Could you check a few things on this model? Use its own coordinates, in mm. Give positions to 0.01 mm unless a question says otherwise; leave off trailing zeros. Loops run counter-clockwise (first coordinate to the right, second up) from the corner with the lowest first, then second, coordinate; pieces in that order, holes last.
1. Imagine slicing it at C-C (x = -2.5). List the corners of the cut face in (y, z) for me, plus the area to 3 significant figures.
2. Imagine slicing it at A-A (x = 0). List the corners of the cut face in (y, z) for me (3 decimals), plus the area to 3 significant figures.
3. Imagine slicing it at B-B (y = 0). List the corners of the cut face in (x, z) for me.
4. For P1, Ø1.7, axis at x = 1.5, y = 0, coming from the -Z side; P2, Ø3, axis at y = -4, z = 3, coming from the -X side; P3, Ø3, axis at x = -2, z = 1.5, coming from the +Y side, each with a flat end and sliding along its axis, tell me the tip position at first contact or that it passes through.
5. I need wall thicknesses on line 1 along X through (y, z) = (0, 2.25); line 2 along X through (y, z) = (3, 12); line 3 along Z through (x, y) = (1.75, -1.5). Which ranges of each line are inside material? Lowest first, please.
```python
from build123d import *

# Parameters (mm, degrees)
F0_R     = 6.35
F1_DEPTH = 12.7
F2_W     = 1.27
F2_H     = 0.508
F2_W_2   = 0.508
F2_H_2   = 1.27
F3_DEPTH = 12.7
F4_R     = 0.254
F6_DEPTH = 10.16
F7_R     = 3.302
F8_DEPTH = 3.175


with BuildPart() as f1:
    # F0 (on Top) → F1 (new body)
    with BuildSketch(Plane.XY):
        Circle(F0_R)
    extrude(amount=F1_DEPTH)

    # F2 (on Top) → F3 (join, through all)
    with BuildSketch(Plane.XY):
        with Locations((0, 6.57217)):
            Rectangle(F2_W, F2_H)
        Polygon((-2.025599, 6.549563), (-3.198926, 6.063555), (-3.004523, 5.594224), (-1.831196, 6.080232), align=None)
        Polygon((-4.377818, 5.275844), (-5.275844, 4.377818), (-4.916634, 4.018608), (-4.018608, 4.916634), align=None)
        Polygon((-6.063555, 3.198926), (-6.549563, 2.025599), (-6.080232, 1.831196), (-5.594224, 3.004523), align=None)
        with Locations((-6.57217, 0)):
            Rectangle(F2_W_2, F2_H_2)
        Polygon((-6.549563, -2.025599), (-6.063555, -3.198926), (-5.594224, -3.004523), (-6.080232, -1.831196), align=None)
        Polygon((-5.275844, -4.377818), (-4.377818, -5.275844), (-4.018608, -4.916634), (-4.916634, -4.018608), align=None)
        Polygon((-3.198926, -6.063555), (-2.025599, -6.549563), (-1.831196, -6.080232), (-3.004523, -5.594224), align=None)
        with Locations((0, -6.57217)):
            Rectangle(F2_W, F2_H)
        Polygon((2.025599, -6.549563), (3.198926, -6.063555), (3.004523, -5.594224), (1.831196, -6.080232), align=None)
        Polygon((4.377818, -5.275844), (5.275844, -4.377818), (4.916634, -4.018608), (4.018608, -4.916634), align=None)
        Polygon((6.063555, -3.198926), (6.549563, -2.025599), (6.080232, -1.831196), (5.594224, -3.004523), align=None)
        with Locations((6.57217, 0)):
            Rectangle(F2_W_2, F2_H_2)
        Polygon((6.549563, 2.025599), (6.063555, 3.198926), (5.594224, 3.004523), (6.080232, 1.831196), align=None)
        Polygon((5.275844, 4.377818), (4.377818, 5.275844), (4.018608, 4.916634), (4.916634, 4.018608), align=None)
        Polygon((3.198926, 6.063555), (2.025599, 6.549563), (1.831196, 6.080232), (3.004523, 5.594224), align=None)
    extrude(amount=F3_DEPTH)

    # F4
    f4_edges = [f1.edges().sort_by_distance(p)[0] for p in [
        (0.635, 6.82617, 6.35),
        (-0.635, 6.82617, 6.35),
        (0.635, 6.31817, 6.35),
        (-0.635, 6.31817, 6.35),
        (1.831196, 6.080232, 6.35),
        (2.025599, 6.549563, 6.35),
        (3.198926, 6.063555, 6.35),
        (3.004523, 5.594224, 6.35),
        (4.377818, 5.275844, 6.35),
        (5.275844, 4.377818, 6.35),
        (4.018608, 4.916634, 6.35),
        (4.916634, 4.018608, 6.35),
        (5.594224, 3.004523, 6.35),
        (6.063555, 3.198926, 6.35),
        (6.549563, 2.025599, 6.35),
        (6.080232, 1.831196, 6.35),
        (6.82617, 0.635, 6.35),
        (6.31817, 0.635, 6.35),
        (6.82617, -0.635, 6.35),
        (6.31817, -0.635, 6.35),
        (6.549563, -2.025599, 6.35),
        (6.080232, -1.831196, 6.35),
        (6.063555, -3.198926, 6.35),
        (5.275844, -4.377818, 6.35),
        (5.594224, -3.004523, 6.35),
        (4.916634, -4.018608, 6.35),
        (4.377818, -5.275844, 6.35),
        (4.018608, -4.916634, 6.35),
        (3.004523, -5.594224, 6.35),
        (3.198926, -6.063555, 6.35),
        (0.635, -6.31817, 6.35),
        (0.635, -6.82617, 6.35),
        (1.831196, -6.080232, 6.35),
        (2.025599, -6.549563, 6.35),
        (-0.635, -6.82617, 6.35),
        (-0.635, -6.31817, 6.35),
        (-1.831196, -6.080232, 6.35),
        (-2.025599, -6.549563, 6.35),
        (-3.198926, -6.063555, 6.35),
        (-3.004523, -5.594224, 6.35),
        (-4.018608, -4.916634, 6.35),
        (-4.377818, -5.275844, 6.35),
        (-5.594224, -3.004523, 6.35),
        (-6.063555, -3.198926, 6.35),
        (-5.275844, -4.377818, 6.35),
        (-4.916634, -4.018608, 6.35),
        (-6.080232, -1.831196, 6.35),
        (-6.549563, -2.025599, 6.35),
        (-6.31817, -0.635, 6.35),
        (-6.82617, -0.635, 6.35),
        (-6.82617, 0.635, 6.35),
        (-6.31817, 0.635, 6.35),
        (-6.080232, 1.831196, 6.35),
        (-6.549563, 2.025599, 6.35),
        (-6.063555, 3.198926, 6.35),
        (-5.594224, 3.004523, 6.35),
        (-4.377818, 5.275844, 6.35),
        (-4.018608, 4.916634, 6.35),
        (-4.916634, 4.018608, 6.35),
        (-5.275844, 4.377818, 6.35),
        (-1.831196, 6.080232, 6.35),
        (-2.025599, 6.549563, 6.35),
        (-3.004523, 5.594224, 6.35),
        (-3.198926, 6.063555, 6.35),
    ]]
    fillet(f4_edges, radius=F4_R)

    # F5 (on Top) → F6 (cut)
    with BuildSketch(Plane.XY):
        with BuildLine():
            Line((2.254026, 2.413), (-2.254026, 2.413))
            ThreePointArc((-2.254026, 2.413), (0, -3.302), (2.254026, 2.413))
        make_face()
    extrude(amount=F6_DEPTH, mode=Mode.SUBTRACT)

    # F7 (on Top) → F8 (cut)
    with BuildSketch(Plane.XY):
        Circle(F7_R)
    extrude(amount=F8_DEPTH, mode=Mode.SUBTRACT)


solid = f1.part
```
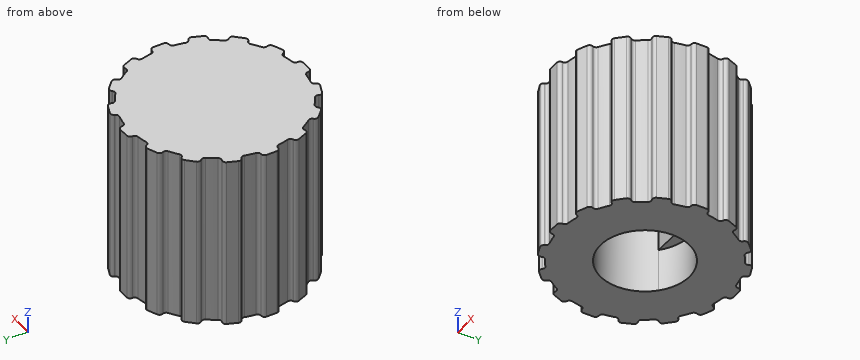
Derived:
1. outline: (-6.35, 0) - (-2.16, 0) - (-2.16, 10.16) - (2.16, 10.16) - (2.16, 0) - (6.35, 0) - (6.35, 12.7) - (-6.35, 12.7) - close
1. area: 118 mm2
2. outline: (-6.826, 0) - (-3.302, 0) - (-3.302, 10.16) - (2.413, 10.16) - (2.413, 3.175) - (3.302, 3.175) - (3.302, 0) - (6.826, 0) - (6.826, 12.7) - (-6.826, 12.7) - close
2. area: 112 mm2
3. outline: (-6.83, 0) - (-3.3, 0) - (-3.3, 10.16) - (3.3, 10.16) - (3.3, 0) - (6.83, 0) - (6.83, 12.7) - (-6.83, 12.7) - close
4. P1: stops at z = 10.16
4. P2: stops at x = -6.35
4. P3: stops at y = 6.8
5. line 1: x = -6.83 to -3.3, 3.3 to 6.83
5. line 2: x = -6.14 to 6.14
5. line 3: z = 10.16 to 12.7
